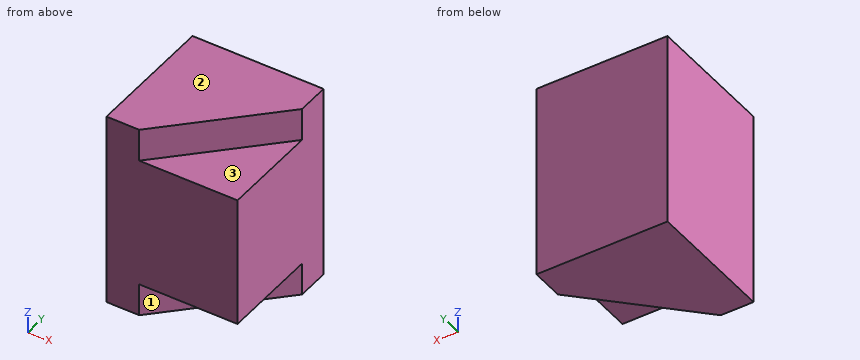
from build123d import *

# Parameters (mm, degrees)
F0_W      = 101.6
F0_H      = 101.6
F1_DEPTH  = 101.6
F3_W      = 101.6
F3_H      = 25.4
F4_DEPTH  = 25.4
F5_W      = 25.4
F5_H      = 76.2
F6_DEPTH  = 25.4
F8_DEPTH  = 25.4
F10_DEPTH = 25.4


with BuildPart() as f1:
    # F0 (on Top) → F1 (new body)
    with BuildSketch(Plane.XY):
        with Locations((50.8, -50.8)):
            Rectangle(F0_W, F0_H)
    extrude(amount=F1_DEPTH)

    # F3 (on face) → F4 (join)
    with BuildSketch(Plane.XY.offset(101.6)):
        with Locations((50.8, -12.7)):
            Rectangle(F3_W, F3_H)
    extrude(amount=F4_DEPTH)

    # F5 (on face) → F6 (join)
    with BuildSketch(Plane.XY.offset(101.6)):
        with Locations((12.7, -63.207563)):
            Rectangle(F5_W, F5_H)
    extrude(amount=F6_DEPTH)

    # F7 (on face) → F8 (join)
    with BuildSketch(Plane.XY.offset(101.6)):
        Polygon((101.6, 0), (0, 0), (0, -101.6), (25.4, -101.6), (25.4, -25.4), (101.6, -25.4), align=None)
        Polygon((25.4, -101.6), (101.6, -25.4), (25.4, -25.4), align=None)
    extrude(amount=F8_DEPTH)

    # F9 (on face) → F10 (join)
    with BuildSketch(Plane(origin=(0, 0, 0), x_dir=(1, 0, 0), z_dir=(0, 0, -1))):
        Polygon((0, 101.6), (0, 0), (101.6, 0), (101.6, 25.4), (25.4, 101.6), align=None)
    extrude(amount=F10_DEPTH)


solid = f1.part
Could you check a few things on this model? Use its own coordinates, in mm. Face numbers are marked on the shaded views. A direction names the side the tool comes from. Round coordinates to 2 decimals unless told otherwise and drop trailing zeros. Loops run counter-clockwise (first coordinate to the right, second up) from the corner with the lowest first, then second, coordinate; pieces in that order, holes last. Notation, with made-up numbers: (-2, -7.75) - (56, -7.75) arc R20 ccw to (56, 25.25) - close; hole circle Ø7 at (-1.5, 87.5). An arc over 180 degrees is marked (long way). Write item = value, one per line.
1) Imagine slicing it at C-C (z = -14). Please give me the cut outline in (x, y), and give its area (3 significant figures).
Computed:
outline = (0, -101.6) - (25.4, -101.6) - (101.6, -25.4) - (101.6, 0) - (0, 0) - close
area = 7,420 mm2
2) I need wall thicknesses on line 1 along Z through (x, y) = (45, -96.5); line 2 along Y through (x, z) = (39.5, -10); line 3 along Y through (x, z) = (57, 118). Which ranges of each line are inside material? Lowest first, please. Write a range as from..to.
Computed:
line_1 = 0..101.6
line_2 = -87.5..0
line_3 = -70..0
3) Imagine slicing it at B-B (y = -71). Please give me the cut outline in (x, z).
Computed:
outline = (0, -25.4) - (56, -25.4) - (56, 0) - (101.6, 0) - (101.6, 101.6) - (56, 101.6) - (56, 127) - (0, 127) - close
4) On a 3-axis mill with a long thin cutter (end or side, diameter ignored), from which of +Z, -Z, +X, -X, +Y, -Y can I reach the whole of each face in a straight line? I mean the marked faces 1, 2 and 3. Say none if no direction works.
Computed:
face_1 = -Z, +X, -Y
face_2 = +Z, +X, -X, +Y, -Y
face_3 = +Z, +X, -Y
5) Imagine slicing it at A-A (x = 40.5). Please give me the cut outline in (y, z), and give its area (3 significant figures).
Computed:
outline = (-101.6, 0) - (-86.5, 0) - (-86.5, -25.4) - (0, -25.4) - (0, 127) - (-86.5, 127) - (-86.5, 101.6) - (-101.6, 101.6) - close
area = 14,700 mm2
6) I'm going to push a flat-ended pin straight in: P1, Ø4, axis at x = 82.5, y = -61.5, coming from the -Z side. Where does the tip first touch, or does it pass through?
Computed:
P1 = 0
